Could you check a few things on this model? Use its own coordinates, in mm. Round coordinates to 2 decimals unless told otherwise and drop trailing zeros. Loops run counter-clockwise (first coordinate to the right, second up) from the corner with the lowest first, then second, coordinate; pieces in that order, holes last. Notation, with made-up numbers: M -13.75,72.25 L 10.25,72.25 A13 cw 10.25,88.25 Z; hole C -13,26 d10. An arc over 180 degrees is marked long. One line per item, written item: value. Start each with the question number.
Q1. I'm going to push flat-ended pins straight in: pin 1 Ø0.9 at (x, y) = (28.5, 2) entering from -Z; pin 2 Ø5 at (x, z) = (2, 7) entering from -Y; pin 3 Ø1.5 at (y, z) = (2, 13.5) entering from +X; pin 4 Ø0.6 at (y, z) = (1, 12.5) entering from -X. Where does each tip first touch, or does it pass through?
Q2. Please list where these lines run through material, in increasing order: line 1 along X through (y, z) = (1.8, 0); line 2 along Z through (x, y) = (5, 2.5); line 3 along Z through (x, y) = (33, 2.95).
Q3. Imagine slicing it at A-A (z = 0). Please give me the cut outline in (x, y).
Q4. Imagine slicing it at C-C (x = 30). Please give me the cut outline in (y, z).
Q5. Imagine slicing it at B-B (x = 20). Please give me the cut outline in (y, z), then the cut area to 3 significant figures.
Q6. Imagine slicing it at D-D (y = 2.5). Give the number of separate pieces and of enclosed holes in the cut face, then the cut area to 3 significant figures.
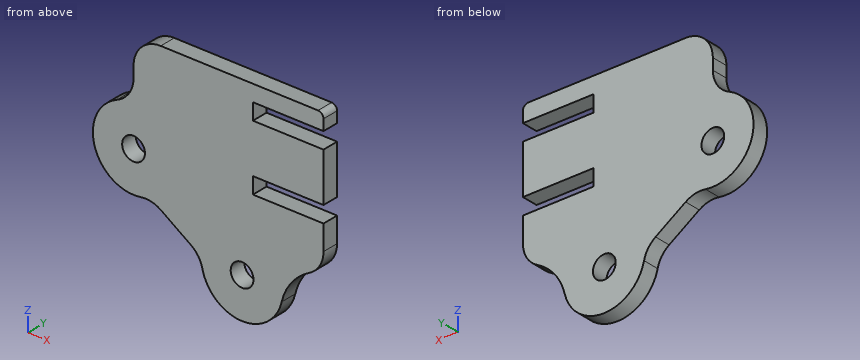
from build123d import *

# Parameters (mm, degrees)
SKETCH1_R           = 2.1
BOSS_EXTRUDE1_DEPTH = 3
FILLET1_R           = 5
SKETCH2_W           = 8
SKETCH2_H           = 3
CUT_EXTRUDE1_DEPTH  = 3
BOSS_EXTRUDE2_DEPTH = 3
FILLET2_R           = 10
SKETCH5_W           = 13
SKETCH5_H           = 3
CUT_EXTRUDE3_DEPTH  = 3.5
FILLET3_R           = 5
FILLET4_R           = 1


with BuildPart() as part:
    # Sketch1 → Boss-Extrude1 (new body)
    with BuildSketch(Plane(origin=(0, 0, 0), x_dir=(1, 0, 0), z_dir=(0, 1, 0))):
        with BuildLine():
            Line((0, -11.456439237), (0, -18.5))
            Line((0, -18.5), (30, -18.5))
            Line((30, -18.5), (30, -10.955880937))
            ThreePointArc((30, -10.955880937), (29.758770483, -9.587800364), (29.064177772, -8.384730498))
            Line((29.064177772, -8.384730498), (22.591994863, -0.671483264))
            ThreePointArc((22.591994863, -0.671483264), (21.491397009, 3.371317526), (23.853330247, 6.832072535))
            ThreePointArc((23.853330247, 6.832072535), (24.386195315, 19.350189707), (12.677699795, 14.889434685))
            ThreePointArc((12.677699795, 14.889434685), (11.918282987, 13.141523465), (10.560020318, 11.804725034))
            Line((10.560020318, 11.804725034), (5.017813295, 8.128440794))
            ThreePointArc((5.017813295, 8.128440794), (3.258028142, 7.396960283), (1.352375582, 7.377064476))
            ThreePointArc((1.352375582, 7.377064476), (-7.172928544, 2.190683933), (-3, -6.873863542))
            ThreePointArc((-3, -6.873863542), (-0.816699867, -8.71782645), (0, -11.456439237))
        make_face()
        with Locations(Location((0, 0, 0), (0, 0, 270))):
            Circle(SKETCH1_R, mode=Mode.SUBTRACT)
        with Locations(Location((20, 13.266499161, 0), (0, 0, 270))):
            Circle(SKETCH1_R, mode=Mode.SUBTRACT)
    extrude(amount=BOSS_EXTRUDE1_DEPTH)

    # Fillet1
    fillet1_edges = [part.edges().sort_by_distance(p)[0] for p in [
        (0, 1.5, 18.5),
    ]]
    fillet(fillet1_edges, radius=FILLET1_R)

    # Sketch2 → Cut-Extrude1 (cut)
    with BuildSketch(Plane(origin=(0, 3, 0), x_dir=(1, 0, 0), z_dir=(0, 1, 0))):
        with Locations((26, -14)):
            Rectangle(SKETCH2_W, SKETCH2_H)
    extrude(amount=-CUT_EXTRUDE1_DEPTH, mode=Mode.SUBTRACT)

    # Sketch4 → Boss-Extrude2 (add)
    with BuildSketch(Plane(origin=(0, 3, 0), x_dir=(1, 0, 0), z_dir=(0, 1, 0))):
        Polygon((27.12691506, 10.930459408), (35, 7.210028784), (35, -0.5), (22, -0.5), (22, -3.5), (35, -3.5), (35, -12.5), (22, -12.5), (22, -15.5), (35, -15.5), (35, -18.5), (18.101899038, -18.5), (15.526805317, 5.265582811), align=None)
    extrude(amount=-BOSS_EXTRUDE2_DEPTH)

    # Fillet2
    fillet2_edges = [part.edges().sort_by_distance(p)[0] for p in [
        (27.12691506, 1.5, -10.930459408),
    ]]
    fillet(fillet2_edges, radius=FILLET2_R)

    # Sketch5 → Cut-Extrude3 (cut)
    with BuildSketch(Plane(origin=(0, 3, 0), x_dir=(1, 0, 0), z_dir=(0, 1, 0))):
        with Locations((28.5, -2)):
            Rectangle(SKETCH5_W, SKETCH5_H)
    extrude(amount=-CUT_EXTRUDE3_DEPTH, mode=Mode.SUBTRACT)

    # Fillet3
    fillet3_edges = [part.edges().sort_by_distance(p)[0] for p in [
        (35, 1.5, -7.210028784),
    ]]
    fillet(fillet3_edges, radius=FILLET3_R)

    # Fillet4
    fillet4_edges = [part.edges().sort_by_distance(p)[0] for p in [
        (35, 1.5, 18.5),
    ]]
    fillet(fillet4_edges, radius=FILLET4_R)


solid = part.part
Report:
1. pin 1: stops at z = -12.9
1. pin 2: stops at y = 0
1. pin 3: stops at x = 22
1. pin 4: stops at x = 0
2. line 1: x = -7.5 to -2.1, 2.1 to 35
2. line 2: z = -8.12 to 18.5
2. line 3: z = -8.06 to 0.5, 3.5 to 12.5, 15.5 to 18.5
3. outline: M -7.5,0 L -2.1,0 L -2.1,3 L -7.5,3 Z; M 2.1,0 L 35,0 L 35,3 L 2.1,3 Z
4. outline: M 0,-10.2 L 3,-10.2 L 3,0.5 L 0,0.5 Z; M 0,3.5 L 3,3.5 L 3,12.5 L 0,12.5 Z; M 0,15.5 L 3,15.5 L 3,18.5 L 0,18.5 Z
5. outline: M 0,-20.77 L 3,-20.77 L 3,-15.37 L 0,-15.37 Z; M 0,-11.17 L 3,-11.17 L 3,18.5 L 0,18.5 Z
5. area: 105 mm²
6. separate pieces: 1
6. enclosed holes: 2
6. area: 1,100 mm²
